```python
from build123d import *

# Parameters (mm, degrees)
F1_DEPTH  = 0.5
F3_DEPTH  = 2
F4_W      = 45
F4_H      = 19.7
F4_W_2    = 43.2
F4_H_2    = 17.7
F5_DEPTH  = 9
F6_W      = 2.5
F6_H      = 2.5
F7_DEPTH  = 3
F8_W      = 7.8
F8_H      = 6
F9_DEPTH  = 0.8
F10_W     = 1.5
F10_H     = 5
F10_H_2   = 5.0084371828
F11_DEPTH = 1
F12_R     = 0.74999
F13_R     = 1


# Not quite as in the source:
# - a fillet or chamfer is up to 0.001 mm smaller than in the source, because OpenCascade refuses the exact size


with BuildPart() as f1:
    # F0 (on Top) → F1 (new body)
    with BuildSketch(Plane.XY):
        with BuildLine():
            Line((0, -15.75), (0, 15.75))
            Line((0, 15.75), (-147, 15.75))
            ThreePointArc((-147, 15.75), (-149.1213203436, 14.8713203436), (-150, 12.75))
            Line((-150, 12.75), (-150, -12.75))
            ThreePointArc((-150, -12.75), (-149.1213203436, -14.8713203436), (-147, -15.75))
            Line((-147, -15.75), (0, -15.75))
        make_face()
        Polygon((45, 19), (0, 19), (0, 15.75), (0, -15.75), (0, -19), (45, -19), align=None)
    extrude(amount=F1_DEPTH)

    # F2 (on face) → F3 (join)
    with BuildSketch(Plane.XY.offset(0.5)):
        Polygon((45, -19), (45, 19), (0, 19), (0, 15.75), (0, -15.75), (0, -19), align=None)
    extrude(amount=F3_DEPTH)

    # F4 (on face) → F5 (join)
    with BuildSketch(Plane.XY.offset(2.5)):
        with Locations((22.5, 0)):
            Rectangle(F4_W, F4_H)
        with Locations((22.6, 0)):
            Rectangle(F4_W_2, F4_H_2, mode=Mode.SUBTRACT)
    extrude(amount=F5_DEPTH)

    # F6 (on face) → F7 (join)
    with BuildSketch(Plane.XY.offset(2.5)):
        with Locations((2.25, 7.6)):
            Rectangle(F6_W, F6_H)
        with Locations((42.95, 7.6)):
            Rectangle(F6_W, F6_H)
        with Locations((42.95, -7.6)):
            Rectangle(F6_W, F6_H)
        with Locations((2.25, -7.6)):
            Rectangle(F6_W, F6_H)
    extrude(amount=F7_DEPTH)

    # F8 (on face) → F9 (cut, through all)
    with BuildSketch(Plane.YZ.offset(45)):
        with Locations((0, 8.5)):
            Rectangle(F8_W, F8_H)
    extrude(amount=-F9_DEPTH, mode=Mode.SUBTRACT)

    # F10 (on face) → F11 (cut, through all)
    with BuildSketch(Plane(origin=(0, 9.85, 0), x_dir=(-1, 0, 0), z_dir=(0, 1, 0))):
        with Locations((-19, 9)):
            Rectangle(F10_W, F10_H)
        with Locations((-6.75, 8.9957814086)):
            Rectangle(F10_W, F10_H_2)
    extrude(amount=-F11_DEPTH, mode=Mode.SUBTRACT)

    # F12 (radius 0.75 in the source; OpenCascade refuses exactly that, so slightly less here)
    f12_edges = [f1.edges().sort_by_distance(p)[0] for p in [
        (18.25, 9.35, 6.5),
        (19.75, 9.35, 6.5),
        (6, 9.35, 6.491563),
        (7.5, 9.35, 6.491563),
    ]]
    fillet(f12_edges, radius=F12_R)

    # F13
    f13_edges = [f1.edges().sort_by_distance(p)[0] for p in [
        (45, 9.85, 7),
        (45, 14.425, 2.5),
        (45, 19, 1.25),
        (22.5, 19, 2.5),
        (0, 14.425, 2.5),
        (0, 9.85, 7),
        (22.5, 9.85, 2.5),
        (0, -9.85, 7),
        (0, -14.425, 2.5),
        (0, -19, 1.25),
        (22.5, -19, 2.5),
        (22.5, -9.85, 2.5),
        (45, -9.85, 7),
        (45, -14.425, 2.5),
        (45, -19, 1.25),
        (0, 19, 1.25),
    ]]
    fillet(f13_edges, radius=F13_R)


solid = f1.part
```
For this review, take the finished solid that the model builds, in its own axes (mm). A direction names the side the tool comes from. Coordinates: 2 decimals unless noted, no trailing zeros. Write each loop counter-clockwise with the first axis right and the second up, starting at its lowest first coordinate (ties: lowest second). Pieces come first, ordered by that corner, then holes. Notation, with made-up numbers: (9, 51) -> (57, 51) arc R25 cw to (57, 82) -> close; hole circle Ø2 at (78.25, 80). An arc over 180 degrees is marked (long way). Put each result on its own line as item: value.
Q1. Take a section at B-B, the plane y = 2. State the section outline as (x, z) points, then the cut area to 3 significant figures.
From the geometry:
outline: (-150, 0) -> (45, 0) -> (45, 5.5) -> (44.2, 5.5) -> (44.2, 2.5) -> (1, 2.5) -> (1, 11.5) -> (0, 11.5) -> (0, 0.5) -> (-150, 0.5) -> close
area: 199 mm2
Q2. The part is to be moulded in two halves that separate along X. For faces 1 (the cylindrical face through (-149.14, -14.85, 0.25)), 2 (the flat face through (22, -9.85, 7)), 3 (the flat face through (22, 8.85, 7)), say which applies: +X half, -X half, draft (parallel to the pull), parting line (faces both ways), or undercut.
From the geometry:
face 1: -X half
face 2: draft
face 3: undercut
Q3. Wall thickness on L1, parallel to X at y = 7, z = 6; L2, parallel to X at y = 7, z = 3.5; L3, parallel to Z at x = -78.5, y = 5.5: over which ranges is each line inside the solid? List them lowest first.
From the geometry:
L1: x = 0 to 1, 44.2 to 45
L2: x = 0 to 3.5, 41.7 to 45
L3: z = 0 to 0.5
Q4. Tool access review of faces 4 (the flat face through (44.2, 0, 5)), 5 (the flat face through (22, -14, 2.5)), 6 (the flat face through (22, 14, 2.5)): name each direction out of +Z, -Z, +X, -X, +Y, -Y from which nothing blocks a thin tool from reaching the whole face with its end or side.
From the geometry:
face 4: +Z
face 5: +Z, +X, -X, -Y
face 6: +Z, +X, -X, +Y
Q5. Take a section at C-C, the plane x = -25. State the section outline as (y, z) points.
From the geometry:
outline: (-15.75, 0) -> (15.75, 0) -> (15.75, 0.5) -> (-15.75, 0.5) -> close
Q6. Clearance check with flat-ended pins moving along their axes: pin 1 Ø1 at (y, z) = (-1, 4.5) entering from -X; pin 2 Ø0.5 at (y, z) = (9.5, 8.5) entering from +X; pin 3 Ø4.5 at (x, z) = (18.5, 6.5) entering from +Y; pin 4 Ø4 at (y, z) = (15, 5.5) entering from -X. State where each tip first meets the part, or that it passes through.
From the geometry:
pin 1: stops at x = 0
pin 2: stops at x = 44.92
pin 3: stops at y = 9.85
pin 4: passes through
Q7. Take a section at A-A, the plane z = 9.5. State the section outline as (x, y) points.
From the geometry:
outline: (0, -8.85) arc R1 ccw to (1, -9.85) -> (44, -9.85) arc R1 ccw to (45, -8.85) -> (45, -3.9) -> (44.2, -3.9) -> (44.2, -8.85) -> (1, -8.85) -> (1, 8.85) -> (6, 8.85) -> (6, 9.85) -> (1, 9.85) arc R1 ccw to (0, 8.85) -> close; (7.5, 8.85) -> (18.25, 8.85) -> (18.25, 9.85) -> (7.5, 9.85) -> close; (19.75, 8.85) -> (44.2, 8.85) -> (44.2, 3.9) -> (45, 3.9) -> (45, 8.85) arc R1 ccw to (44, 9.85) -> (19.75, 9.85) -> close
